```python
from build123d import *

# Parameters (mm, degrees)
F0_W     = 100
F0_H     = 100
F1_DEPTH = 2
F2_DEPTH = 50
F3_R     = 3.5
F4_DEPTH = 104.001


with BuildPart() as f1:
    # F0 (on Top) → F1 (new body)
    with BuildSketch(Plane.XY):
        with BuildLine():
            ThreePointArc((-49.1308821316, -52), (0, -71.5391052434), (49.1308821316, -52))
            Line((49.1308821316, -52), (-49.1308821316, -52))
        make_face()
        Rectangle(F0_W, F0_H)
        with BuildLine():
            Line((-49.1308821316, 52), (49.1308821316, 52))
            ThreePointArc((49.1308821316, 52), (0, 71.5391052434), (-49.1308821316, 52))
        make_face()
        with BuildLine():
            Line((49.1308821316, 52), (52, 52))
            ThreePointArc((52, 52), (0, 73.5391052434), (-52, 52))
            Line((-52, 52), (-49.1308821316, 52))
            ThreePointArc((-49.1308821316, 52), (0, 71.5391052434), (49.1308821316, 52))
        make_face()
        with BuildLine():
            ThreePointArc((50, 51.1648666472), (49.5671999408, 51.5842637735), (49.1308821316, 52))
            Line((49.1308821316, 52), (-49.1308821316, 52))
            ThreePointArc((-49.1308821316, 52), (-49.5671999408, 51.5842637735), (-50, 51.1648666472))
            Line((-50, 51.1648666472), (-50, 50))
            Line((-50, 50), (50, 50))
            Line((50, 50), (50, 51.1648666472))
        make_face()
        with BuildLine():
            Line((-49.1308821316, 52), (-52, 52))
            Line((-52, 52), (-52, 49.1308821316))
            ThreePointArc((-52, 49.1308821316), (-51.010138926, 50.1578439107), (-50, 51.1648666472))
            ThreePointArc((-50, 51.1648666472), (-49.5671999408, 51.5842637735), (-49.1308821316, 52))
        make_face()
        with BuildLine():
            Line((52, 49.1308821316), (52, 52))
            Line((52, 52), (49.1308821316, 52))
            ThreePointArc((49.1308821316, 52), (49.5671999408, 51.5842637735), (50, 51.1648666472))
            ThreePointArc((50, 51.1648666472), (51.010138926, 50.1578439107), (52, 49.1308821316))
        make_face()
        with BuildLine():
            Line((49.1308821316, -52), (52, -52))
            Line((52, -52), (52, -49.1308821316))
            ThreePointArc((52, -49.1308821316), (51.010138926, -50.1578439107), (50, -51.1648666472))
            ThreePointArc((50, -51.1648666472), (49.5671999408, -51.5842637735), (49.1308821316, -52))
        make_face()
        with BuildLine():
            ThreePointArc((-52, -52), (0, -73.5391052434), (52, -52))
            Line((52, -52), (49.1308821316, -52))
            ThreePointArc((49.1308821316, -52), (0, -71.5391052434), (-49.1308821316, -52))
            Line((-49.1308821316, -52), (-52, -52))
        make_face()
        with BuildLine():
            Line((-52, -49.1308821316), (-52, -52))
            Line((-52, -52), (-49.1308821316, -52))
            ThreePointArc((-49.1308821316, -52), (-49.5671999408, -51.5842637735), (-50, -51.1648666472))
            ThreePointArc((-50, -51.1648666472), (-51.010138926, -50.1578439107), (-52, -49.1308821316))
        make_face()
        with BuildLine():
            ThreePointArc((-50, 51.1648666472), (-51.010138926, 50.1578439107), (-52, 49.1308821316))
            Line((-52, 49.1308821316), (-52, -49.1308821316))
            ThreePointArc((-52, -49.1308821316), (-51.010138926, -50.1578439107), (-50, -51.1648666472))
            Line((-50, -51.1648666472), (-50, -50))
            Line((-50, -50), (-50, 50))
            Line((-50, 50), (-50, 51.1648666472))
        make_face()
        with BuildLine():
            Line((52, -49.1308821316), (52, 49.1308821316))
            ThreePointArc((52, 49.1308821316), (51.010138926, 50.1578439107), (50, 51.1648666472))
            Line((50, 51.1648666472), (50, 50))
            Line((50, 50), (50, -50))
            Line((50, -50), (50, -51.1648666472))
            ThreePointArc((50, -51.1648666472), (51.010138926, -50.1578439107), (52, -49.1308821316))
        make_face()
        with BuildLine():
            Line((-49.1308821316, -52), (49.1308821316, -52))
            ThreePointArc((49.1308821316, -52), (49.5671999408, -51.5842637735), (50, -51.1648666472))
            Line((50, -51.1648666472), (50, -50))
            Line((50, -50), (-50, -50))
            Line((-50, -50), (-50, -51.1648666472))
            ThreePointArc((-50, -51.1648666472), (-49.5671999408, -51.5842637735), (-49.1308821316, -52))
        make_face()
    extrude(amount=F1_DEPTH)

    # F0 (on Top) → F2 (join)
    with BuildSketch(Plane.XY):
        with BuildLine():
            ThreePointArc((-50, 51.1648666472), (-51.010138926, 50.1578439107), (-52, 49.1308821316))
            Line((-52, 49.1308821316), (-52, -49.1308821316))
            ThreePointArc((-52, -49.1308821316), (-51.010138926, -50.1578439107), (-50, -51.1648666472))
            Line((-50, -51.1648666472), (-50, -50))
            Line((-50, -50), (-50, 50))
            Line((-50, 50), (-50, 51.1648666472))
        make_face()
        with BuildLine():
            Line((-49.1308821316, 52), (-52, 52))
            Line((-52, 52), (-52, 49.1308821316))
            ThreePointArc((-52, 49.1308821316), (-51.010138926, 50.1578439107), (-50, 51.1648666472))
            ThreePointArc((-50, 51.1648666472), (-49.5671999408, 51.5842637735), (-49.1308821316, 52))
        make_face()
        with BuildLine():
            Line((49.1308821316, 52), (52, 52))
            ThreePointArc((52, 52), (0, 73.5391052434), (-52, 52))
            Line((-52, 52), (-49.1308821316, 52))
            ThreePointArc((-49.1308821316, 52), (0, 71.5391052434), (49.1308821316, 52))
        make_face()
        with BuildLine():
            Line((52, -49.1308821316), (52, 49.1308821316))
            ThreePointArc((52, 49.1308821316), (51.010138926, 50.1578439107), (50, 51.1648666472))
            Line((50, 51.1648666472), (50, 50))
            Line((50, 50), (50, -50))
            Line((50, -50), (50, -51.1648666472))
            ThreePointArc((50, -51.1648666472), (51.010138926, -50.1578439107), (52, -49.1308821316))
        make_face()
        with BuildLine():
            Line((52, 49.1308821316), (52, 52))
            Line((52, 52), (49.1308821316, 52))
            ThreePointArc((49.1308821316, 52), (49.5671999408, 51.5842637735), (50, 51.1648666472))
            ThreePointArc((50, 51.1648666472), (51.010138926, 50.1578439107), (52, 49.1308821316))
        make_face()
        with BuildLine():
            Line((49.1308821316, -52), (52, -52))
            Line((52, -52), (52, -49.1308821316))
            ThreePointArc((52, -49.1308821316), (51.010138926, -50.1578439107), (50, -51.1648666472))
            ThreePointArc((50, -51.1648666472), (49.5671999408, -51.5842637735), (49.1308821316, -52))
        make_face()
        with BuildLine():
            ThreePointArc((-52, -52), (0, -73.5391052434), (52, -52))
            Line((52, -52), (49.1308821316, -52))
            ThreePointArc((49.1308821316, -52), (0, -71.5391052434), (-49.1308821316, -52))
            Line((-49.1308821316, -52), (-52, -52))
        make_face()
        with BuildLine():
            Line((-52, -49.1308821316), (-52, -52))
            Line((-52, -52), (-49.1308821316, -52))
            ThreePointArc((-49.1308821316, -52), (-49.5671999408, -51.5842637735), (-50, -51.1648666472))
            ThreePointArc((-50, -51.1648666472), (-51.010138926, -50.1578439107), (-52, -49.1308821316))
        make_face()
    extrude(amount=F2_DEPTH)

    # F3 (on face) → F4 (cut, through all)
    with BuildSketch(Plane.YZ.offset(52)):
        with Locations((0, 20)):
            Circle(F3_R)
    extrude(amount=-F4_DEPTH, mode=Mode.SUBTRACT)


solid = f1.part
```
Design review of the part built by this model. Coordinates are the model's own, in mm. A direction names the side the tool comes from. Coordinates: 2 decimals unless noted, no trailing zeros. Loops run counter-clockwise (first coordinate to the right, second up) from the corner with the lowest first, then second, coordinate; pieces in that order, holes last. Notation, with made-up numbers: M -17,-30 L 4,-30 A25 ccw 4,3 Z; hole C 38,81.25 d8. An arc over 180 degrees is marked long. One line per question, with ' | ' between items.
(1) We need section C-C (y = 49). Give the boundary of the cut face in (x, z), and give its area (3 significant figures).
Filled in:
outline: M -52,0 L 52,0 L 52,50 L 50,50 L 50,2 L -50,2 L -50,50 L -52,50 Z | area: 400 mm^2
(2) For pin 1 Ø8 at (y, z) = (53, 19.5) entering from -X; pin 2 Ø6 at (x, y) = (8, -20) entering from +Z; pin 3 Ø1 at (y, z) = (-53, 31.5) entering from +X; pin 4 Ø12 at (x, z) = (-12.5, 34) entering from +Y, all flat-tipped, find the tip position at first contact; note any pin that passes through.
Filled in:
pin 1: stops at x = -52 | pin 2: stops at z = 2 | pin 3: stops at x = 51.5 | pin 4: stops at y = 73.25
(3) Machinability: for faces 4 (the face through (-50.3, 5.8, 50)), 5 (the face through (50, 1, 26)), which of the approach directions +Z, -Z, +X, -X, +Y, -Y give a long, thin tool a straight path to every point of the face, cutting with its end or side? Answer none if there is none.
Filled in:
face 4: +Z, +X, -X, +Y, -Y | face 5: +Z
(4) We need section D-D (z = 45). Give the boundary of the cut face in (x, y).
Filled in:
outline: M -52,-52 A73.54 ccw 52,-52 L 52,52 A73.54 ccw -52,52 Z; hole M -50,-51.16 A71.54 ccw 50,-51.16 L 50,51.16 A71.54 ccw -50,51.16 Z
(5) We need section B-B (y = 0). Give the boundary of the cut face in (x, z).
Filled in:
outline: M -52,0 L 52,0 L 52,16.5 L 50,16.5 L 50,2 L -50,2 L -50,16.5 L -52,16.5 Z; M -52,23.5 L -50,23.5 L -50,50 L -52,50 Z; M 50,23.5 L 52,23.5 L 52,50 L 50,50 Z
(6) Wall thickness on probe 1 along X at (y, z) = (37, 32); probe 2 along Z at (x, y) = (-51, 0); probe 3 along Z at (x, y) = (14.5, 31): over which ranges is each line inside the solid? List them lowest first.
Filled in:
probe 1: x = -52 to -50, 50 to 52 | probe 2: z = 0 to 16.5, 23.5 to 50 | probe 3: z = 0 to 2
(7) We need section A-A (z = 20). Give the boundary of the cut face in (x, y).
Filled in:
outline: M -52,-52 A73.54 ccw 52,-52 L 52,-3.5 L 50,-3.5 L 50,-51.16 A71.54 cw -50,-51.16 L -50,-3.5 L -52,-3.5 Z; M -52,3.5 L -50,3.5 L -50,51.16 A71.54 cw 50,51.16 L 50,3.5 L 52,3.5 L 52,52 A73.54 ccw -52,52 Z
(8) Draft analysis for pull direction X (two halves, no side actions). For faces 1 (the face through (-1, 1, 0)), 2 (the face through (-0.809, -73.535, 24.65)), 3 (the face through (-50, -1, 26)), state which applies: released by +X, released by -X, zero draft, split by the parting line, or undercut.
Filled in:
face 1: zero draft | face 2: split by the parting line | face 3: undercut
